Autodesk Inventor part; units mm, degrees
ref_plane "YZ Plane" through (0, 0, 0) normal (1, 0, 0) x (0, 1, 0)
ref_plane "XZ Plane" through (0, 0, 0) normal (0, 1, 0) x (-1, 0, 0)
ref_plane "XY Plane" through (0, 0, 0) normal (0, 0, 1) x (1, 0, 0)
sketch "Sketch1" plane through (0, 0, 0) normal (1, 0, 0) x (0, 1, 0)
  arc A0 (17.2522, 102.4526) -> (0, 107) centre (0, 72) ccw
  arc A1 (0, -47) -> (29.2642, -36.7778) centre (0, 0) ccw
  arc A2 (56.3935, 52.3189) -> (59.948, 78.2643) centre (53, 66) ccw
  arc A3 (61.6337, -11.0214) -> (56.3309, 13.511) centre (52.9167, -0.0663) ccw
  line L0 (17.2522, 102.4526) -> (59.948, 78.2643)
  line L1 (61.6337, -11.0214) -> (29.2642, -36.7778)
  arc A4 (56.3935, 52.3189) -> (56.3309, 13.511) centre (61.2084, 32.9071) ccw
  arc A5 (21, 72) -> (0, 93) centre (0, 72) ccw
  arc A6 (0, -32.5) -> (21, 24.8042) centre (0, 0) ccw
  line L2 (21, 72) -> (21, 30.8042)
  circle A7 centre (53, 66) radius 7.5
  circle A8 centre (52.9167, -0.0663) radius 7.5
  arc A9 (-56.3704, 13.5882) -> (-56.3704, 52.4118) centre (-61.1854, 33) ccw
  line L3 (-20.9781, 66) -> (-21, 24.8042)
  circle A10 centre (-53, 66) radius 7.5
  line L4 (-28.9912, 91.6089) -> (-58.5472, 78.8541)
  arc A11 (0, 107) -> (-28.9912, 91.6089) centre (0, 72) ccw
  arc A12 (-58.5472, 78.8541) -> (-56.3704, 52.4118) centre (-53, 66) ccw
  arc A13 (-56.3704, 13.5882) -> (-61.717, -10.9551) centre (-53, 0) ccw
  arc A14 (-21, 24.8042) -> (0, -32.5) centre (0, 0) ccw
  arc A15 (-29.2642, -36.7778) -> (0, -47) centre (0, 0) ccw
  line L5 (-61.717, -10.9551) -> (-29.2642, -36.7778)
  circle A16 centre (-53, 0) radius 7.5
  arc A17 (0, 93) -> (-20.9781, 71.0401) centre (0, 72) ccw
  line L6 (21, 30.8042) -> (21, 24.8042)
  line L7 (-20.9781, 71.0401) -> (-20.9781, 66)
  dimension "d15" = 15
  dimension "d16" = 20
  dimension "d17" = 32.5
  dimension "d18" = 47
  dimension "d19" = 21
  dimension "d20" = 72
  dimension "d21" = 106
  dimension "d22" = 66
  dimension "d23" = 15
extrude "Extrusion1" add sketch "Sketch1" against normal mid plane 20
properties part number "hw9"
Build history of the part. All positions in model axes, mm. A direction names the side the tool comes from. Give positions to 0.01 mm unless a question says otherwise; leave off trailing zeros. Loops run counter-clockwise (first coordinate to the right, second up) from the corner with the lowest first, then second, coordinate; pieces in that order, holes last. Notation, with made-up numbers: (-32, -5) - (-28, -5) arc R7 cw to (-28, 8) - close; hole circle Ø1 at (55, 29). An arc over 180 degrees is marked (long way). Write item = value, one per line. Start each with the question number.
1) Pull direction Z, two halves, no side cores. Call faces 3 (the flat face through (0.1, -45.7, -23.7)), 4 (the cylindrical face through (0.14, -30.7, -10.66)), 5 (the flat face through (10, -31, 31)), 6 (the cylindrical face through (0.14, -16.2, 103.025)): +Z half, -Z half, draft (parallel to the pull), parting line (faces both ways), or undercut.
2) Tool access for faces 1 (the cylindrical face through (0.14, 66.645, 2.678)), 2 (the cylindrical face through (-0.14, 30.7, -10.66)): list every direction of +Z, -Z, +X, -X, +Y, -Y with a clear straight run to the whole face (end or side of a thin tool).
3) Band-saw the part on B-B on z = 76. Give the cut face in (x, y), plus the area to 3 significant figures.
4) Band-saw the part on A-A on y = -27. Give the cut face in (x, z).
5) Band-saw the part on D-D on y = -53. Give the cut face in (x, z), plus the area to 3 significant figures.
6) Drop flat-ended pins along their axis: pin 1 Ø4 at (x, z) = (1, 10) entering from -Y; pin 2 Ø12 at (x, y) = (-2, 26) entering from +Z; pin 3 Ø4 at (x, z) = (-6, -30) entering from +Y; pin 4 Ø12 at (y, z) = (-53, 66) entering from +X. Give the stop position or say it passes through.
7) Probe probe 1 along Z at (x, y) = (-3.75, -53); probe 2 along Y at (x, z) = (-8, 32); probe 3 along Z at (x, y) = (0.75, 47). List the from-to ranges inside material, lowest first. Write a range as from..to.
8) Band-saw the part on C-C on z = -4.5. Give the cut face in (x, y).
Final values:
q1.face_3 = -Z half
q1.face_4 = undercut
q1.face_5 = draft
q1.face_6 = +Z half
q2.face_1 = +X, -X, +Y
q2.face_2 = +X, -X
q3.outline = (-10, -62.8) - (10, -62.8) - (10, -20.62) - (-10, -20.62) - close; (-10, 20.62) - (10, 20.62) - (10, 62.93) - (-10, 62.93) - close
q3.area = 1,690 mm²
q4.outline = (-10, -38.47) - (10, -38.47) - (10, -18.09) - (-10, -18.09) - close; (-10, 18.09) - (10, 18.09) - (10, 94.27) - (-10, 94.27) - close
q5.outline = (-10, -17.89) - (10, -17.89) - (10, -7.5) - (-10, -7.5) - close; (-10, 7.5) - (10, 7.5) - (10, 14.75) - (-10, 14.75) - close; (-10, 51.25) - (10, 51.25) - (10, 58.5) - (-10, 58.5) - close; (-10, 73.5) - (10, 73.5) - (10, 81.25) - (-10, 81.25) - close
q5.area = 653 mm²
q6.pin_1 = -64.49
q6.pin_2 = 100.9
q6.pin_3 = 40.3
q6.pin_4 = through
q7.probe_1 = -17.89..-7.5, 7.5..14.75, 51.25..58.5, 73.5..81.25
q7.probe_2 = -41.21..-21, 21..41.23
q7.probe_3 = -22.67..-4.68, 4.54..18.83, 46.98..61.5, 70.5..85.6
q8.outline = (-10, -66.26) - (10, -66.26) - (10, -59) - (-10, -59) - close; (-10, -47) - (10, -47) - (10, -32.19) - (-10, -32.19) - close; (-10, 32.19) - (10, 32.19) - (10, 46.87) - (-10, 46.87) - close; (-10, 58.97) - (10, 58.97) - (10, 66.2) - (-10, 66.2) - close
